Print and shaded views of the part. All mm, measured from the part's lowest x, y and z. Coordinates: 2 decimals unless noted, no trailing zeros. Loops run counter-clockwise (first coordinate to the right, second up) from the corner with the lowest first, then second, coordinate; pieces in that order, holes last. Notation, with made-up numbers: M -12,29.25 L 11,29.25 A10 cw 11,45.25 Z; hole C 28.5,22.5 d5. An arc over 180 degrees is marked long. Use a Markdown table: item, result. Add a question column.
1) Band-saw the part on D-D (z = 65.5). List the corners of the cut face in (x, y).
2) Band-saw the part on C-C (x = 43). List the corners of the cut face in (y, z).
3) Band-saw the part on B-B (z = 6). List the corners of the cut face in (x, y).
4) Band-saw the part on A-A (y = 30). List the corners of the cut face in (x, z), plus the area to 3 significant figures.
5) Pull direction Z, two halves, no side cores. Call the marked faces 1, 2 and 3: released by +Z, released by -Z, zero draft, split by the parting line, or undercut.
6) Wall check: probe 1 along Y at (x, z) = (30, 73.5); probe 2 along Z at (x, y) = (5.5, 20.5); probe 3 along X at (y, z) = (25.5, 8.5). Give the ranges that are in metal, low to high. Write a range as from..to.
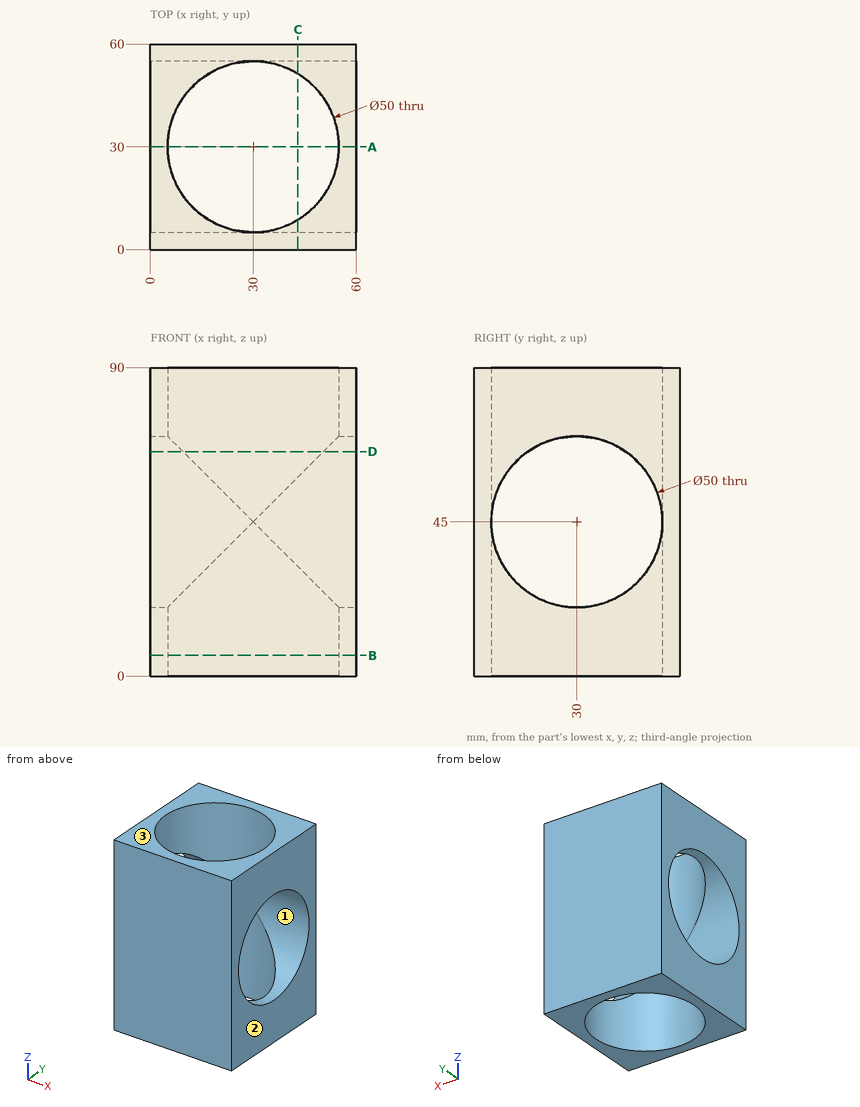
Entries:
| question | item | result |
|---|---|---|
| 1 | outline | M 0,0 L 60,0 L 60,15.69 L 50.5,15.69 A25 cw 9.5,15.69 L 0,15.69 Z; M 0,44.31 L 9.5,44.31 A25 cw 50.5,44.31 L 60,44.31 L 60,60 L 0,60 Z |
| 2 | outline | M 0,0 L 8.65,0 L 8.65,32 A25 cw 8.65,58 L 8.65,90 L 0,90 Z; M 51.35,0 L 60,0 L 60,90 L 51.35,90 L 51.35,58 A25 cw 51.35,32 Z |
| 3 | outline | M 0,0 L 60,0 L 60,60 L 0,60 Z; hole C 30,30 d50 |
| 4 | outline | M 0,0 L 5,0 L 5,20 L 0,20 Z; M 0,70 L 5,70 L 5,90 L 0,90 Z; M 55,0 L 60,0 L 60,20 L 55,20 Z; M 55,70 L 60,70 L 60,90 L 55,90 Z |
| 4 | area | 400 mm2 |
| 5 | face 1 | undercut |
| 5 | face 2 | zero draft |
| 5 | face 3 | released by +Z |
| 6 | probe 1 | 0..5, 55..60 |
| 6 | probe 2 | 0..21.88, 68.12..90 |
| 6 | probe 3 | 0..5.41, 54.59..60 |
